Job drawing, mm, ordinate dimensions from the low corner. One solid piece. A direction names the side the tool comes from. Round coordinates to 2 decimals unless told otherwise and drop trailing zeros. Write each loop counter-clockwise with the first axis right and the second up, starting at its lowest first coordinate (ties: lowest second). Pieces come first, ordered by that corner, then holes. Notation, with made-up numbers: (17, 15.5) -> (75, 15.5) arc R11 cw to (75, 20.5) -> close; hole circle Ø5 at (41, -32.5). An arc over 180 degrees is marked (long way). Use CSV: the item, a comma, the result in double quotes. Start each with the question number.
(1) Drop flat-ended pins along their axis: pin 1 (3 mm diameter, centred on x = 58.5, z = 3.5, fed in from -Y); pin 2 (5 mm diameter, centred on y = 30.5, z = 5, fed in from +X); pin 3 (5 mm diameter, centred on x = 13, z = 6.5, fed in from +Y). Give the stop position or say it passes through.
(2) Probe line 1 (Y direction, x = 22, z = 5.5); line 2 (Y direction, x = 3.5, z = 5.5); line 3 (Y direction, x = 41.5, z = 5.75). List the from-to ranges inside material, lowest first. Write a range as [from, to].
(3) Saw through at A-A (x = 47). Give the cut face in (y, z).
(4) Saw through at C-C (y = 74). Give the cut face in (x, z), plus the area to 3 significant figures.
(5) Which spindle directions (+Z, -Z, +X, -X, +Y, -Y) get a long thin tool onto all of the face, cutting with end or side? Do the marked faces 1, 2, 3, 4 and 5. Say none if no direction does.
(6) Saw through at D-D (x = 34.5). Give the cut face in (y, z), plus the area to 3 significant figures.
(7) Saw through at B-B (z = 8.75). Give the cut face in (x, y), plus the area to 3 significant figures.
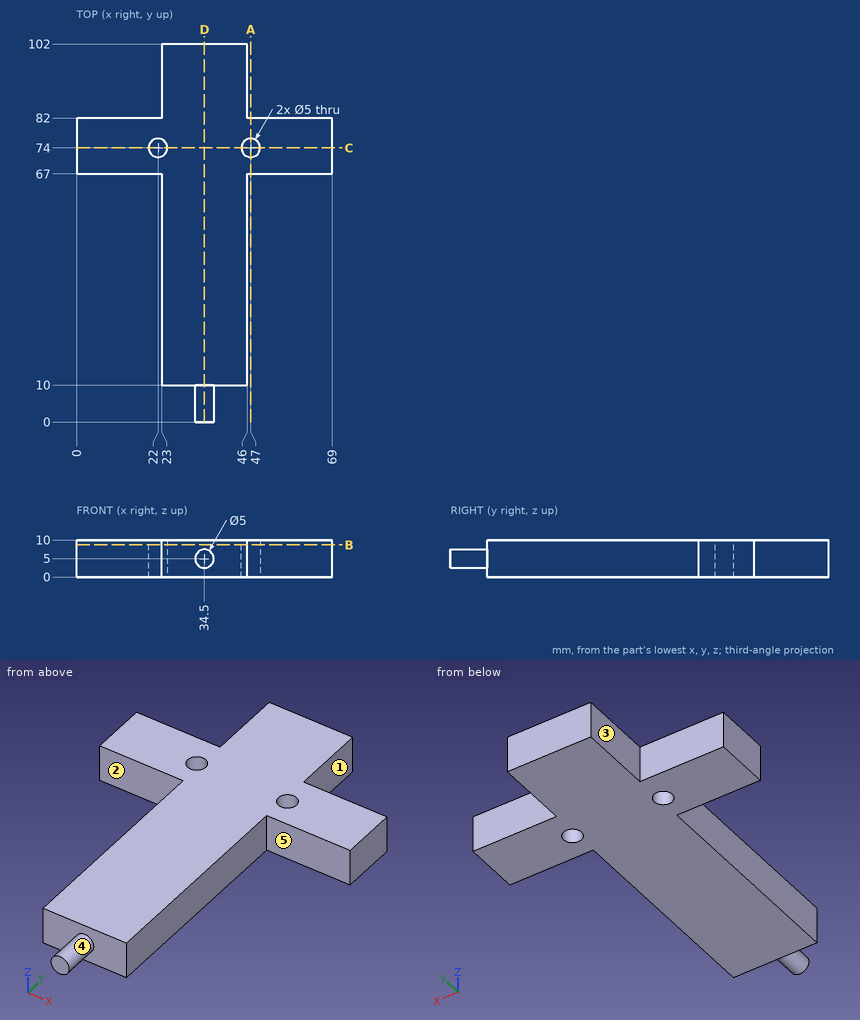
Answers:
1,pin 1,"stops at y = 67"
1,pin 2,"stops at x = 46"
1,pin 3,"stops at y = 82"
2,line 1,"y = [67, 71.5], [76.5, 82]"
2,line 2,"y = [67, 82]"
2,line 3,"y = [10, 102]"
3,outline,"(67, 0) -> (71.5, 0) -> (71.5, 10) -> (67, 10) -> close; (76.5, 0) -> (82, 0) -> (82, 10) -> (76.5, 10) -> close"
4,outline,"(0, 0) -> (19.5, 0) -> (19.5, 10) -> (0, 10) -> close; (24.5, 0) -> (44.5, 0) -> (44.5, 10) -> (24.5, 10) -> close; (49.5, 0) -> (69, 0) -> (69, 10) -> (49.5, 10) -> close"
4,area,"590 mm²"
5,face 1,"+Z, -Z, +X, +Y"
5,face 2,"+Z, -Z, -X, -Y"
5,face 3,"+Z, -Z, -X, +Y"
5,face 4,"-Y"
5,face 5,"+Z, -Z, +X, -Y"
6,outline,"(0, 2.5) -> (10, 2.5) -> (10, 0) -> (102, 0) -> (102, 10) -> (10, 10) -> (10, 7.5) -> (0, 7.5) -> close"
6,area,"970 mm²"
7,outline,"(0, 67) -> (23, 67) -> (23, 10) -> (46, 10) -> (46, 67) -> (69, 67) -> (69, 82) -> (46, 82) -> (46, 102) -> (23, 102) -> (23, 82) -> (0, 82) -> close; hole circle Ø5 at (22, 74); hole circle Ø5 at (47, 74)"
7,area,"2,770 mm²"
